Verification items for the finished model (mm, model axes). A direction names the side the tool comes from. Give positions to 0.01 mm unless a question says otherwise; leave off trailing zeros. Write each loop counter-clockwise with the first axis right and the second up, starting at its lowest first coordinate (ties: lowest second). Pieces come first, ordered by that corner, then holes. Notation, with made-up numbers: (54.25, 27) - (64.25, 27) arc R34 cw to (64.25, 61) - close; hole circle Ø5 at (28.5, 64.25). An arc over 180 degrees is marked (long way). Put each result on its own line as item: value.
from build123d import *

# Parameters (mm, degrees)
SKETCH1_W            = 1000
SKETCH1_H            = 700
SKETCH1_W_2          = 900
SKETCH1_H_2          = 600
BOSS_EXTRUDE1_DEPTH  = 150
SKETCH2_W            = 100
SKETCH2_H            = 600
CUT_EXTRUDE1_DEPTH   = 1000
SKETCH3_R            = 50
BOSS_EXTRUDE2_DEPTH  = 600
BOSS_EXTRUDE3_START  = -180
BOSS_EXTRUDE3_DEPTH  = 180
SKETCH5_W            = 100
SKETCH5_H            = 100
BOSS_EXTRUDE4_DEPTH  = 600
SKETCH7_R            = 47
BOSS_EXTRUDE15_DEPTH = 600
BOSS_EXTRUDE16_DEPTH = 115


with BuildPart() as part:
    # Sketch1 → Boss-Extrude1 (new body)
    with BuildSketch(Plane.XY):
        Rectangle(SKETCH1_W, SKETCH1_H)
        Rectangle(SKETCH1_W_2, SKETCH1_H_2, mode=Mode.SUBTRACT)
    extrude(amount=BOSS_EXTRUDE1_DEPTH)

    # Sketch2 → Cut-Extrude1 (cut)
    with BuildSketch(Plane(origin=(500, 0, 0), x_dir=(0, 0, -1), z_dir=(1, 0, 0))):
        with Locations((-100, 0)):
            Rectangle(SKETCH2_W, SKETCH2_H)
    extrude(amount=-CUT_EXTRUDE1_DEPTH, mode=Mode.SUBTRACT)

    # Sketch3 → Boss-Extrude2 (add)
    with BuildSketch(Plane.XZ.offset(-300)):
        with Locations(Location((460, 110, 0), (0, 0, 126.869897646))):
            Circle(SKETCH3_R)
    boss_extrude2 = extrude(amount=BOSS_EXTRUDE2_DEPTH)

    # Mirror1: Boss-Extrude2 across plane
    add(boss_extrude2.mirror(Plane(origin=(0, 0, 0), x_dir=(0, 0, 1), z_dir=(1, 0, 0))))

    # Sketch4 → Boss-Extrude3 (add)
    with BuildSketch(Plane.XZ.offset(300).offset(BOSS_EXTRUDE3_START)):
        with BuildLine():
            Line((-460, 162), (460, 162))
            ThreePointArc((460, 162), (512, 110), (460, 58))
            Line((460, 58), (-460, 58))
            ThreePointArc((-460, 58), (-512, 110), (-460, 162))
        make_face()
        with BuildLine():
            Line((-460, 160), (460, 160))
            ThreePointArc((460, 160), (510, 110), (460, 60))
            Line((460, 60), (-460, 60))
            ThreePointArc((-460, 60), (-510, 110), (-460, 160))
        make_face(mode=Mode.SUBTRACT)
    boss_extrude3 = extrude(amount=BOSS_EXTRUDE3_DEPTH)

    # Mirror2: Boss-Extrude3 across plane
    add(boss_extrude3.mirror(Plane.ZX))

    # Sketch5 → Boss-Extrude4 (add)
    with BuildSketch(Plane(origin=(0, 0, 0), x_dir=(-1, 0, 0), z_dir=(0, 0, -1))):
        with Locations((-450, 300)):
            Rectangle(SKETCH5_W, SKETCH5_H)
        with Locations((450, 300)):
            Rectangle(SKETCH5_W, SKETCH5_H)
        with Locations((450, -300)):
            Rectangle(SKETCH5_W, SKETCH5_H)
        with Locations((-450, -300)):
            Rectangle(SKETCH5_W, SKETCH5_H)
    extrude(amount=BOSS_EXTRUDE4_DEPTH)

    # Sketch7 → Boss-Extrude15 (add)
    with BuildSketch(Plane.XZ.offset(-300)):
        with Locations(Location((-212, 110, 0), (0, 0, 121.672433426))):
            Circle(SKETCH7_R)
    boss_extrude15 = extrude(amount=BOSS_EXTRUDE15_DEPTH)

    # Sketch10 → Boss-Extrude16 (add, symmetric)
    with BuildSketch(Plane(origin=(0, 0, 0), x_dir=(1, 0, 0), z_dir=(0, 1, 0))):
        with BuildLine():
            Line((-211.988019901, -158.999998535), (-456.82601912, -161.903042737))
            ThreePointArc((-456.82601912, -161.903042737), (-512, -110), (-456.82601912, -58.096957263))
            Line((-456.82601912, -58.096957263), (-211.988019901, -61.000001465))
            ThreePointArc((-211.988019901, -61.000001465), (-163, -110), (-211.988019901, -158.999998535))
        make_face()
        with BuildLine():
            Line((-212, -157), (-456.899440499, -159.903772711))
            ThreePointArc((-456.899440499, -159.903772711), (-510, -110), (-456.899440499, -60.096227289))
            Line((-456.899440499, -60.096227289), (-212, -63))
            ThreePointArc((-212, -63), (-165, -110), (-212, -157))
        make_face(mode=Mode.SUBTRACT)
    boss_extrude16 = extrude(amount=BOSS_EXTRUDE16_DEPTH, both=True)

    # Mirror3: Boss-Extrude15, Boss-Extrude16 across plane
    add(boss_extrude15.mirror(Plane(origin=(0, 0, 0), x_dir=(0, 0, 1), z_dir=(1, 0, 0))))
    add(boss_extrude16.mirror(Plane(origin=(0, 0, 0), x_dir=(0, 0, 1), z_dir=(1, 0, 0))))


solid = part.part
Q1. Scan lines: line 1 along X through (y, z) = (280, -515); line 2 along Y through (x, z) = (102, 56); line 3 along Z through (x, y) = (124, -221.5). Record each from-to range of solid material in increasing order.
Answers follow:
line 1: x = -500 to -400, 400 to 500
line 2: y = -350 to -300, 300 to 350
line 3: z = 58 to 60, 160 to 162
Q2. Section check C-C, the plane z = -350.5. Record the cut outline in (x, y).
Answers follow:
outline: (-500, -350) - (-400, -350) - (-400, -250) - (-500, -250) - close; (-500, 250) - (-400, 250) - (-400, 350) - (-500, 350) - close; (400, -350) - (500, -350) - (500, -250) - (400, -250) - close; (400, 250) - (500, 250) - (500, 350) - (400, 350) - close
Q3. Section check B-B, the plane y = -92. Record the cut outline in (x, z), plus the area to 3 significant figures.
Answers follow:
outline: (-500, 0) - (-450, 0) - (-450, 50) - (-500, 50) - close; (-456.83, 58.1) - (-211.99, 61) arc R49 ccw to (-211.99, 159) - (-456.83, 161.9) arc R52 ccw (long way) to start; (211.99, 61) - (456.83, 58.1) arc R52 ccw (long way) to (456.83, 161.9) - (211.99, 159) arc R49 ccw to start; (450, 0) - (500, 0) - (500, 50) - (450, 50) - close; hole (-456.9, 60.1) - (-212, 63) arc R47 cw to (-212, 157) - (-456.9, 159.9) arc R50 cw to start; hole (212, 63) - (456.9, 60.1) arc R50 cw to (456.9, 159.9) - (212, 157) arc R47 cw to start
area: 37,800 mm2
Q4. Set-up check for faces 4 (the face through (-475, -4, 50)), 5 (the face through (451, -250, -296)), 6 (the face through (-375, 115, 160)): record each of +Z, -Z, +X, -X, +Y, -Y from which the full face is reachable in a straight line by a thin tool's end or side.
Answers follow:
face 4: +X, -X
face 5: -Z, +X, -X
face 6: none
Q5. Release check for a two-part mould opening along Z. For faces 1 (the face through (6, -300, 106)), 2 (the face through (-7, -350, 20)), 3 (the face through (451, 301, -600)) record: released by +Z, released by -Z, zero draft, split by the parting line, or undercut.
Answers follow:
face 1: undercut
face 2: zero draft
face 3: released by -Z
Q6. Go/stop test with flat-tipped pins: pin 1 Ø8 at (x, y) = (351.5, -201) entering from -Z; pin 2 Ø2 at (x, z) = (-208, 155) entering from +Y; pin 3 Ø6 at (x, z) = (-81, 158) entering from -Y; pin 4 Ø4 at (x, y) = (-62.5, -116.5) entering from +Z. Record where each tip stops, or that it passes through.
Answers follow:
pin 1: stops at z = 58
pin 2: stops at y = 300
pin 3: stops at y = -300
pin 4: passes through
Q7. Section check D-D, the plane x = -46. Record the cut outline in (y, z).
Answers follow:
outline: (-350, 0) - (-300, 0) - (-300, 58) - (-120, 58) - (-120, 60) - (-300, 60) - (-300, 150) - (-350, 150) - close; (-300, 160) - (-120, 160) - (-120, 162) - (-300, 162) - close; (120, 58) - (300, 58) - (300, 0) - (350, 0) - (350, 150) - (300, 150) - (300, 60) - (120, 60) - close; (120, 160) - (300, 160) - (300, 162) - (120, 162) - close
Q8. Section check A-A, the plane y = 286. Record the cut outline in (x, z).
Answers follow:
outline: (-500, -600) - (-400, -600) - (-400, 0) - (-450, 0) - (-450, 50) - (-500, 50) - close; (-460, 58) - (460, 58) arc R52 ccw to (460, 162) - (-460, 162) arc R52 ccw to start; circle Ø94 at (-212, 110); circle Ø94 at (212, 110); (400, -600) - (500, -600) - (500, 50) - (450, 50) - (450, 0) - (400, 0) - close; hole (-460, 60) - (460, 60) arc R50 cw to (460, 160) - (-460, 160) arc R50 cw to start
